Could you check a few things on this model? Use its own coordinates, in mm. A direction names the side the tool comes from. Round coordinates to 2 decimals unless told otherwise and drop trailing zeros. Write each loop counter-clockwise with the first axis right and the second up, starting at its lowest first coordinate (ties: lowest second). Pieces come first, ordered by that corner, then holes. Notation, with made-up numbers: (64, 41.5) -> (79, 41.5) arc R34 cw to (79, 76.5) -> close; hole circle Ø11 at (67.25, -28). An arc over 180 degrees is marked (long way). Answer in a Markdown table with one row per item.
from build123d import *

# Parameters (mm, degrees)
SKETCH1_W           = 50
SKETCH1_H           = 50
BOSS_EXTRUDE1_DEPTH = 300
CUT_EXTRUDE2_REACH  = 304.076
SKETCH3_W           = 22
SKETCH3_H           = 41


with BuildPart() as part:
    # Sketch1 → Boss-Extrude1 (new body)
    with BuildSketch(Plane(origin=(0, 0, 0), x_dir=(0, 0, -1), z_dir=(1, 0, 0))):
        Rectangle(SKETCH1_W, SKETCH1_H)
    extrude(amount=BOSS_EXTRUDE1_DEPTH)

    # Sketch3 → Cut-Extrude2 (cut, up to next)
    with BuildSketch(Plane.ZY, mode=Mode.PRIVATE) as cut_extrude2_sk1:
        Rectangle(SKETCH3_W, SKETCH3_H)
    cut_extrude2_tool1 = extrude(cut_extrude2_sk1.sketch, amount=-CUT_EXTRUDE2_REACH, mode=Mode.PRIVATE) & part.part
    add(cut_extrude2_tool1.solids().sort_by_distance((0, 0, 0))[0], mode=Mode.SUBTRACT)


solid = part.part
1) Imagine slicing it at B-B, the plane z = -1.5. Please give me the cut outline in (x, y).
Findings:
| item | result |
|---|---|
| outline | (0, -25) -> (300, -25) -> (300, -20.5) -> (0, -20.5) -> close; (0, 20.5) -> (300, 20.5) -> (300, 25) -> (0, 25) -> close |
2) Imagine slicing it at C-C, the plane x = 111. Please give me the cut outline in (y, z), plus the area to 3 significant figures.
Findings:
| item | result |
|---|---|
| outline | (-25, -25) -> (25, -25) -> (25, 25) -> (-25, 25) -> close; hole (-20.5, -11) -> (20.5, -11) -> (20.5, 11) -> (-20.5, 11) -> close |
| area | 1,600 mm^2 |
3) For faces 4 (the face through (148, 0, 25)), 5 (the face through (148, 0, -11)), which set-ups out of +Z, -Z, +X, -X, +Y, -Y let a thin tool reach every point of the face, with its end or its side?
Findings:
| item | result |
|---|---|
| face 4 | +Z, +X, -X, +Y, -Y |
| face 5 | +X, -X |
4) Imagine slicing it at A-A, the plane y = 9.5. Please give me the cut outline in (x, z), plus the area to 3 significant figures.
Findings:
| item | result |
|---|---|
| outline | (0, -25) -> (300, -25) -> (300, -11) -> (0, -11) -> close; (0, 11) -> (300, 11) -> (300, 25) -> (0, 25) -> close |
| area | 8,400 mm^2 |
5) Thinking about a two-plate mould opening in Y: for faces 1 (the face through (148, 0, -25)), 2 (the face through (148, 20.5, 0)), 3 (the face through (148, -25, 0)), which applies, +Y half, -Y half, draft (parallel to the pull), parting line (faces both ways), or undercut?
Findings:
| item | result |
|---|---|
| face 1 | draft |
| face 2 | undercut |
| face 3 | -Y half |
6) Please list where these lines run through material, in increasing order: line 1 (Z direction, x = 228, y = -12); line 2 (Y direction, x = 257, z = -7.5).
Findings:
| item | result |
|---|---|
| line 1 | z = -25 to -11, 11 to 25 |
| line 2 | y = -25 to -20.5, 20.5 to 25 |
7) For pin 1 (4 mm diameter, centred on y = -13, z = -11.5, fed in from -X), with a flat end and sliding along its axis, tell me the tip position at first contact or that it passes through.
Findings:
| item | result |
|---|---|
| pin 1 | stops at x = 0 |
